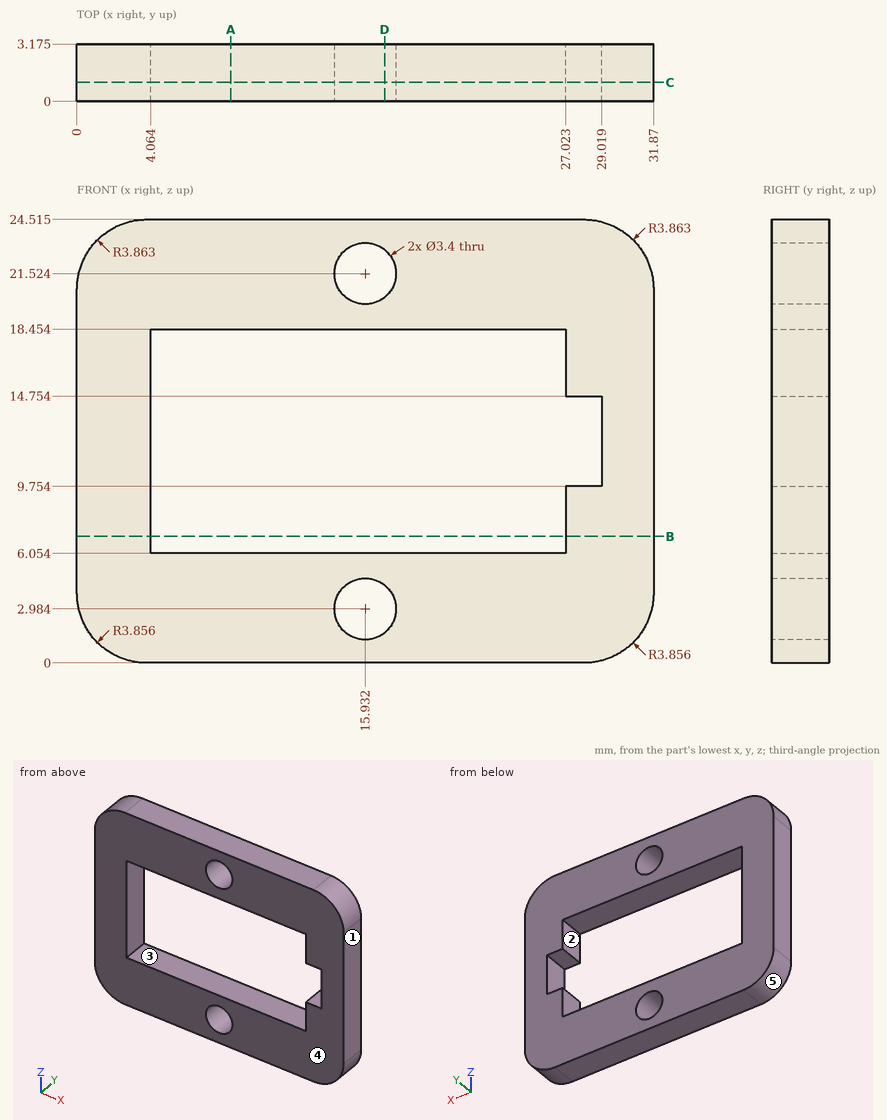
Source: three-view drawing plus pictorial views. Frame: mm from the lowest corner of the part. A direction names the side the tool comes from. Give positions to 0.01 mm unless a question says otherwise; leave off trailing zeros. Loops run counter-clockwise (first coordinate to the right, second up) from the corner with the lowest first, then second, coordinate; pieces in that order, holes last. Notation, with made-up numbers: M 56.25,57 L 85.25,57 A9 ccw 85.25,62 Z; hole C 19,54 d11. An arc over 180 degrees is marked long. Use CSV: the item, a comma, the result in double quotes.
(1) Set-up query: the marked faces 1 and 2. Return all of +Z, -Z, +X, -X, +Y, -Y with unobstructed straight access to the full face (end or side cutting, diameter ignored); none if empty.
Outcome:
face 1,"+Z, -Z, +X, +Y, -Y"
face 2,"+Y, -Y"
(2) Pull-direction query (X, two-part tool) for the marked faces 3, 4 and 5; classes: pulls with the +X half, pulls with the -X half, needs draft (parallel to the pull), parting line crosses it, or undercut.
Outcome:
face 3,"undercut"
face 4,"needs draft"
face 5,"pulls with the -X half"
(3) Section C-C, the plane y = 1.05. Return loops of the section in (x, z) (1 decimal).
Outcome:
outline,"M 0,3.9 A3.9 ccw 3.9,0 L 28,0 A3.9 ccw 31.9,3.9 L 31.9,20.7 A3.9 ccw 28,24.5 L 3.9,24.5 A3.9 ccw 0,20.7 Z; hole M 4.1,6.1 L 27,6.1 L 27,9.8 L 29,9.8 L 29,14.8 L 27,14.8 L 27,18.5 L 4.1,18.5 Z; hole C 15.9,3 d3.4; hole C 15.9,21.5 d3.4"
(4) Material intervals for L1, parallel to Z at x = 22.5, y = 2.45 (1 decimal); L2, parallel to Z at x = 27.5, y = 0.55 (1 decimal); L3, parallel to X at y = 2.65, z = 6.25, sorted ascending. Write a range as [from, to].
Outcome:
L1,"z = [0, 6.1], [18.5, 24.5]"
L2,"z = [0, 9.8], [14.8, 24.5]"
L3,"x = [0, 4.06], [27.02, 31.87]"
(5) Pin query (flat end, axial travel): P1, Ø3, axis at x = 15.93, z = 2.98, coming from the -Y side. Return the tip coordinate at first contact, or that it passes through.
Outcome:
P1,"passes through"
(6) Section D-D, the plane x = 17. Return loops of the section in (y, z) (1 decimal).
Outcome:
outline,"M 0,0 L 3.2,0 L 3.2,1.7 L 0,1.7 Z; M 0,4.3 L 3.2,4.3 L 3.2,6.1 L 0,6.1 Z; M 0,18.5 L 3.2,18.5 L 3.2,20.2 L 0,20.2 Z; M 0,22.8 L 3.2,22.8 L 3.2,24.5 L 0,24.5 Z"
(7) Section A-A, the plane x = 8.5. Return loops of the section in (y, z) (1 decimal).
Outcome:
outline,"M 0,0 L 3.2,0 L 3.2,6.1 L 0,6.1 Z; M 0,18.5 L 3.2,18.5 L 3.2,24.5 L 0,24.5 Z"
(8) Section B-B, the plane z = 7. Return loops of the section in (x, y) (1 decimal).
Outcome:
outline,"M 0,0 L 4.1,0 L 4.1,3.2 L 0,3.2 Z; M 27,0 L 31.9,0 L 31.9,3.2 L 27,3.2 Z"
